from build123d import *

# Parameters (mm, degrees)
SKETCH1_W           = 150
SKETCH1_H           = 50
BOSS_EXTRUDE1_DEPTH = 160
FILLET2_R           = 50
SHELL1_T            = -2
CUT_EXTRUDE1_DEPTH  = 2
SKETCH20_W          = 2
SKETCH20_H          = 100
BOSS_EXTRUDE2_DEPTH = 5
SKETCH21_W          = 80
SKETCH21_H          = 2
CUT_EXTRUDE2_DEPTH  = 1
SKETCH22_W          = 80
SKETCH22_H          = 2
CUT_EXTRUDE3_DEPTH  = 1


with BuildPart() as part:
    # Sketch1 → Boss-Extrude1 (new body)
    with BuildSketch(Plane(origin=(0, 0, 0), x_dir=(0, 0, -1), z_dir=(1, 0, 0))):
        Rectangle(SKETCH1_W, SKETCH1_H)
    extrude(amount=-BOSS_EXTRUDE1_DEPTH)

    # Fillet2
    fillet2_edges = [part.edges().sort_by_distance(p)[0] for p in [
        (-80, 25, -75),
    ]]
    fillet(fillet2_edges, radius=FILLET2_R - 0.0001)  # a hair under: the kernel refuses the full size

    # Shell1
    shell1_openings = [part.faces().sort_by_distance(p)[0] for p in [
        (-80, 0, 75),
    ]]
    offset(amount=SHELL1_T, openings=shell1_openings, kind=Kind.INTERSECTION)

    # Sketch17 → Cut-Extrude1 (cut)
    with BuildSketch(Plane(origin=(0, 25, 0), x_dir=(1, 0, 0), z_dir=(0, 1, 0))):
        Polygon((-80, 25), (-158, 25), (-158, -75), (-2, -75), (-2, 25), align=None)
    extrude(amount=-CUT_EXTRUDE1_DEPTH, mode=Mode.SUBTRACT)

    # Sketch20 → Boss-Extrude2 (add)
    with BuildSketch(Plane(origin=(0, 25, 0), x_dir=(1, 0, 0), z_dir=(0, 1, 0))):
        with Locations((-159, -25)):
            Rectangle(SKETCH20_W, SKETCH20_H)
        with Locations((-1, -25)):
            Rectangle(SKETCH20_W, SKETCH20_H)
    extrude(amount=BOSS_EXTRUDE2_DEPTH)

    # Sketch21 → Cut-Extrude2 (cut)
    with BuildSketch(Plane(origin=(-158, 0, 0), x_dir=(0, 0, -1), z_dir=(1, 0, 0))):
        with Locations((-15, 26)):
            Rectangle(SKETCH21_W, SKETCH21_H)
    extrude(amount=-CUT_EXTRUDE2_DEPTH, mode=Mode.SUBTRACT)

    # Sketch22 → Cut-Extrude3 (cut)
    with BuildSketch(Plane.ZY.offset(2)):
        with Locations((15, 26)):
            Rectangle(SKETCH22_W, SKETCH22_H)
    extrude(amount=-CUT_EXTRUDE3_DEPTH, mode=Mode.SUBTRACT)

    # Sketch25 → Cut-Revolve1 (revolve, cut)
    with BuildSketch(Plane(origin=(0, 25, 0), x_dir=(1, 0, 0), z_dir=(0, 1, 0))):
        with BuildLine():
            ThreePointArc((-1.475259699, -50.499387542), (-1.999387542, -50.024740301), (-1.524740301, -49.500612458))
            Line((-1.524740301, -49.500612458), (-1.5, -50))
            Line((-1.5, -50), (-1.475259699, -50.499387542))
        make_face()
    revolve(axis=Axis((-1.5, 25, 50), (-0.049480602249094376, 0, -0.9987750847919)), mode=Mode.SUBTRACT)

    # Sketch26 → Cut-Revolve2 (revolve, cut)
    with BuildSketch(Plane(origin=(0, 25, 0), x_dir=(1, 0, 0), z_dir=(0, 1, 0))):
        with BuildLine():
            Line((-158, -51.676352911), (-159, -51.676352911))
            ThreePointArc((-159, -51.676352911), (-158.5, -52.176352911), (-158, -51.676352911))
        make_face()
    revolve(axis=Axis((-158, 25, 51.676352911), (-1, 0, 0)), mode=Mode.SUBTRACT)


solid = part.part
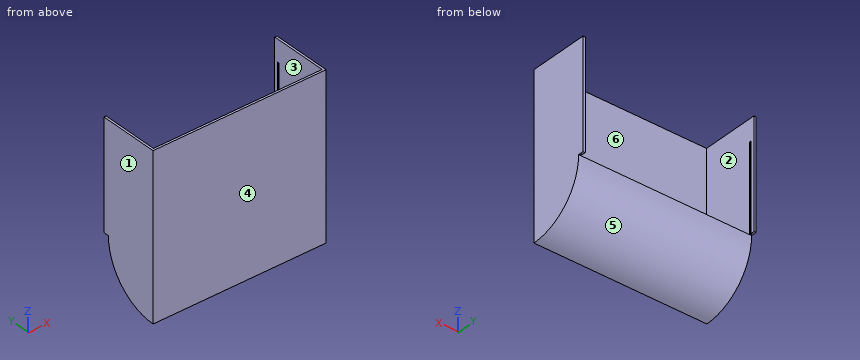
Verification items for the finished model (mm, model axes). Face numbers are marked on the shaded views. A direction names the side the tool comes from. Round coordinates to 2 decimals unless told otherwise and drop trailing zeros. Loops run counter-clockwise (first coordinate to the right, second up) from the corner with the lowest first, then second, coordinate; pieces in that order, holes last. Notation, with made-up numbers: (-22.75, 64.25) - (35.25, 64.25) arc R28 cw to (35.25, 96.25) - close; hole circle Ø7 at (45, 58.25). An arc over 180 degrees is marked (long way). Use a Markdown table: item, result. Add a question column.
1. Release check for a two-part mould opening along Y. For the marked faces 1, 2, 3 and 4 record: released by +Y, released by -Y, zero draft, split by the parting line, or undercut.
2. Thickness scan on probe 1 along X at (y, z) = (-1.5, 27.5); probe 2 along Y at (x, z) = (-121, 36); probe 3 along Y at (x, z) = (-79, -67). Record the ranges inside material, lowest first. Write a range as [from, to].
3. Section check A-A, the plane z = 65. Record the boundary of the cut face in (x, y).
4. Section check D-D, the plane y = -4.5. Record the boundary of the cut face in (x, z).
5. Section check B-B, the plane z = -44. Record the boundary of the cut face in (x, y), plus the area to 3 significant figures.
6. Access from +Z, -Z, +X, -X, +Y, -Y to the whole of each face (thin tool, end or side, straight path). Record for the marked faces 5 and 6.
7. Gauge pin test, flat ends, axial feed: pin 1 (1.6 mm diameter, centred on x = -1, y = 27.5, fed in from -Z); pin 2 (6 mm diameter, centred on x = -59, y = 9.5, fed in from -Z); pin 3 (1 mm diameter, centred on x = -50.5, y = 23.5, fed in from +Z). Record the tip position at first contact, or that the pin passes through.
Checks:
| question | item | result |
|---|---|---|
| 1 | face 1 | zero draft |
| 1 | face 2 | undercut |
| 1 | face 3 | undercut |
| 1 | face 4 | released by -Y |
| 2 | probe 1 | x = [-160, -158], [-2, 0] |
| 2 | probe 2 | y = [-25, -23] |
| 2 | probe 3 | y = [-25, -23], [-1.76, 2.13] |
| 3 | outline | (-160, -25) - (0, -25) - (0, 30) - (-2, 30) - (-2, -23) - (-158, -23) - (-158, 30) - (-160, 30) - close |
| 4 | outline | (-160, -70.6) - (0, -70.6) - (0, 75) - (-2, 75) - (-2, -68.4) - (-158, -68.4) - (-158, 75) - (-160, 75) - close |
| 5 | outline | (-160, -25) - (0, -25) - (0, 21.25) - (-160, 21.25) - close; hole (-158, -23) - (-2, -23) - (-2, 19.08) - (-158, 19.08) - close |
| 5 | area | 835 mm^2 |
| 6 | face 5 | -Z, +X, -X, +Y |
| 6 | face 6 | +Z |
| 7 | pin 1 | stops at z = -25 |
| 7 | pin 2 | stops at z = -63.83 |
| 7 | pin 3 | stops at z = -25 |
